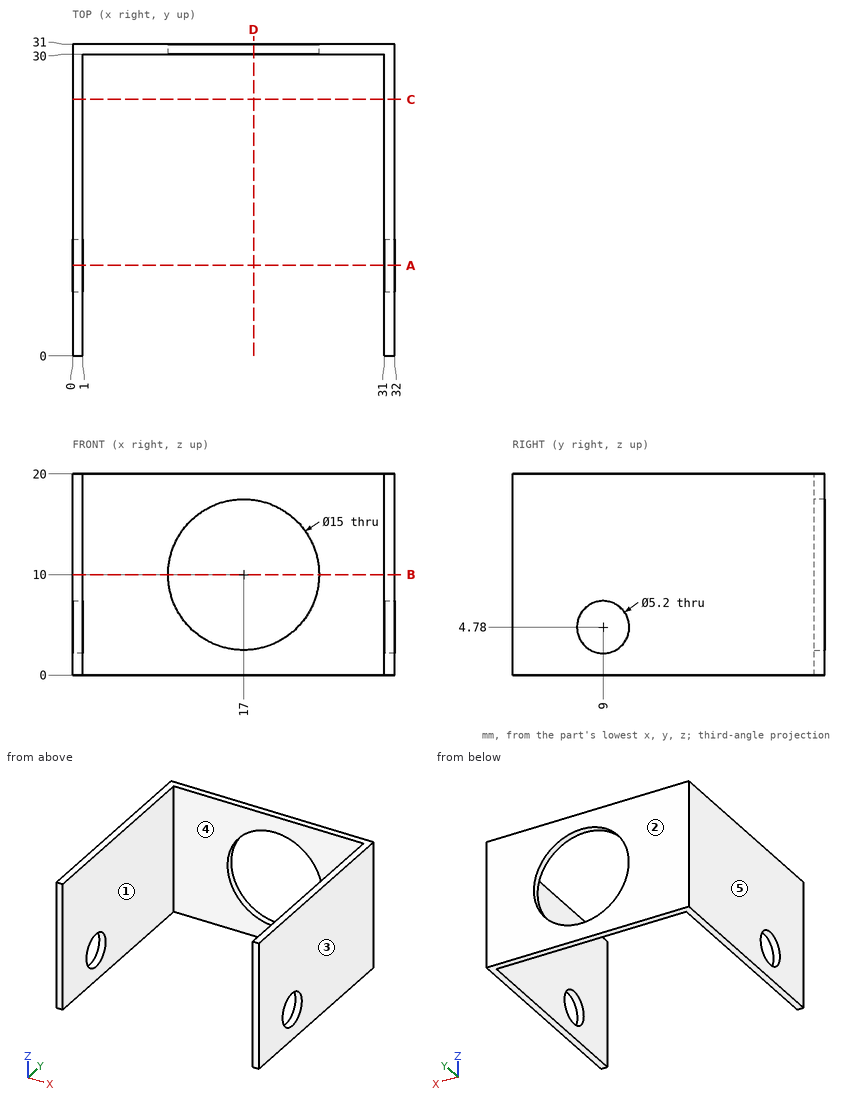
Geometry: see drawing. Coordinates: mm, zero at the bounding-box minimum. A direction names the side the tool comes from. Round coordinates to 2 decimals unless told otherwise and drop trailing zeros. Order: outer loops, then holes, each group sorted by start corner. A loop starts at its lowest first (then second) coordinate and runs counter-clockwise, first axis right, second up. Notation, with made-up numbers: (88, -27) -> (100, -27) arc R24 ccw to (100, -10) -> close; hole circle Ø1 at (-3, 19). An arc over 180 degrees is marked (long way). Write each question's results on one line, items separated by ' | '.
Q1. Section query A-A (y = 9). Output: boundary loops of the cut face in (x, z), and give its area (3 significant figures).
Response values:
outline: (0, 0) -> (1, 0) -> (1, 2.18) -> (0, 2.18) -> close; (0, 7.38) -> (1, 7.38) -> (1, 20) -> (0, 20) -> close; (31, 0) -> (32, 0) -> (32, 2.18) -> (31, 2.18) -> close; (31, 7.38) -> (32, 7.38) -> (32, 20) -> (31, 20) -> close | area: 29.6 mm²
Q2. Ray query, line 1 along X through (y, z) = (20.5, 1.5); line 2 along X through (y, z) = (30.75, 10); line 3 along Y through (x, z) = (3, 2). Return the intervals inside material, ascending.
Response values:
line 1: 0 to 1, 31 to 32 | line 2: 0 to 9.5, 24.5 to 32 | line 3: 30 to 31
Q3. Pin query (flat end, axial travel): pin 1 Ø2 at (x, z) = (5.5, 16.5) entering from -Y. Return the tip coordinate at first contact, or that it passes through.
Response values:
pin 1: y = 30
Q4. Pull-direction query (X, two-part tool) for the marked faces 3, 4 and 5; classes: released by +X, released by -X, zero draft, split by the parting line, or undercut.
Response values:
face 3: released by +X | face 4: undercut | face 5: released by -X
Q5. Access query for the marked faces 1 and 2. Directions: +Z, -Z, +X, -X, +Y, -Y. A direction counts if a zero-diameter tool reaches every point of the face in a straight line with its end or side. Return the directions, or none.
Response values:
face 1: +Z, -Z, -Y | face 2: +Z, -Z, +X, -X, +Y
Q6. Section query C-C (y = 25.5). Output: boundary loops of the cut face in (x, z), and give its area (3 significant figures).
Response values:
outline: (0, 0) -> (1, 0) -> (1, 20) -> (0, 20) -> close; (31, 0) -> (32, 0) -> (32, 20) -> (31, 20) -> close | area: 40.0 mm²
Q7. Section query D-D (x = 18). Output: boundary loops of the cut face in (y, z).
Response values:
outline: (30, 0) -> (31, 0) -> (31, 2.57) -> (30, 2.57) -> close; (30, 17.43) -> (31, 17.43) -> (31, 20) -> (30, 20) -> close
Q8. Section query B-B (z = 10). Output: boundary loops of the cut face in (x, y).
Response values:
outline: (0, 0) -> (1, 0) -> (1, 30) -> (9.5, 30) -> (9.5, 31) -> (0, 31) -> close; (24.5, 30) -> (31, 30) -> (31, 0) -> (32, 0) -> (32, 31) -> (24.5, 31) -> close
